```python
from build123d import *

# Parameters (mm, degrees)
F0_R          = 2.5
F1_DEPTH      = 10
F2_R          = 9
F3_DEPTH      = 18
F5_START      = -4
F4_R          = 4
F5_DEPTH      = 21.4
F6_R          = 1.5
F7_DEPTH      = 25.4
F7_DEPTH_BACK = 32.004


with BuildPart() as f1:
    # F0 (on Front) → F1 (new body)
    with BuildSketch(Plane.XZ):
        Circle(F0_R)
    extrude(amount=F1_DEPTH)

    # F2 (on Front) → F3 (join)
    with BuildSketch(Plane.XZ):
        Circle(F2_R)
    extrude(amount=-F3_DEPTH)

    # F4 (on Front) → F5 (cut)
    with BuildSketch(Plane.XZ.offset(F5_START)):
        Circle(F4_R)
    extrude(amount=-F5_DEPTH, mode=Mode.SUBTRACT)

    # F6 (on Right) → F7 (cut, two sides)
    with BuildSketch(Plane.YZ) as f7_sk:
        with Locations((15.5, 0)):
            Circle(F6_R)
    extrude(amount=-F7_DEPTH, mode=Mode.SUBTRACT)
    extrude(f7_sk.sketch, amount=F7_DEPTH_BACK, mode=Mode.SUBTRACT)


solid = f1.part
```
The listing builds one solid part. Answer for the finished solid, in the listing's coordinates (mm). A direction names the side the tool comes from. Round coordinates to 2 decimals unless told otherwise and drop trailing zeros. Loops run counter-clockwise (first coordinate to the right, second up) from the corner with the lowest first, then second, coordinate; pieces in that order, holes last.
1) A cutting plane is placed at B-B on x = 0. Determine the outline of the cut face in (y, z).
Outcome:
outline: (-10, -2.5) - (0, -2.5) - (0, -9) - (18, -9) - (18, -4) - (4, -4) - (4, 4) - (18, 4) - (18, 9) - (0, 9) - (0, 2.5) - (-10, 2.5) - close
2) For faces 4 (the face through (2, 0, -2)), 5 (the face through (3.695, 10.902, -1.532)), 6 (the face through (6.317, 15.175, -1.464)), determine the directions among +Z, -Z, +X, -X, +Y, -Y from which every point of the face is accessible in a straight line to the end or side of a thin tool.
Outcome:
face 4: -Y
face 5: +Y
face 6: +X, -X
3) For a pull along Y with two mould halves and no side action, classify faces 1 (the face through (0, -10, 0)), 2 (the face through (4, 18, -2)), 3 (the face through (-6.317, 15.175, -1.464)) as released by +Y, released by -Y, zero draft, split by the parting line, or undercut.
Outcome:
face 1: released by -Y
face 2: released by +Y
face 3: undercut
4) Given P1, Ø1.5, axis at x = -7, y = -1, coming from the +Z side; P2, Ø6, axis at y = 8.5, z = -6, coming from the -X side; P3, Ø10, axis at x = 5.5, z = 6, coming from the -Y side; P4, Ø5, axis at y = -0.5, z = 1.5, coming from the +X side, each flat-ended and moving along its own axis, determine where each tip first touches the part or whether it passes through.
Outcome:
P1: passes through
P2: stops at x = -8.49
P3: stops at y = 0
P4: stops at x = 9
5) A cutting plane is placed at A-A on z = 0. Determine the outline of the cut face in (x, y), plus the area to 3 significant figures.
Outcome:
outline: (-9, 0) - (-2.5, 0) - (-2.5, -10) - (2.5, -10) - (2.5, 0) - (9, 0) - (9, 14) - (4, 14) - (4, 4) - (-4, 4) - (-4, 14) - (-9, 14) - close; (-9, 17) - (-4, 17) - (-4, 18) - (-9, 18) - close; (4, 17) - (9, 17) - (9, 18) - (4, 18) - close
area: 232 mm2
6) A cutting plane is placed at D-D on y = -4.5. Determine the outline of the cut face in (x, z), plus the area to 3 significant figures.
Outcome:
outline: circle Ø5 at (0, 0)
area: 19.6 mm2
7) A cutting plane is placed at C-C on y = 15.5. Determine the outline of the cut face in (x, z), plus the area to 3 significant figures.
Outcome:
outline: (-8.87, -1.5) arc R9 ccw to (8.87, -1.5) - (3.71, -1.5) arc R4 cw to (-3.71, -1.5) - close; (-8.87, 1.5) - (-3.71, 1.5) arc R4 cw to (3.71, 1.5) - (8.87, 1.5) arc R9 ccw to start
area: 174 mm2
8) Consider line 1 (Z direction, x = 0, y = 14); line 2 (Y direction, x = 7.35, z = 0). Determine where each line is inside the solid, lowest interval first.
Outcome:
line 1: z = -9 to -4, 4 to 9
line 2: y = 0 to 14, 17 to 18
